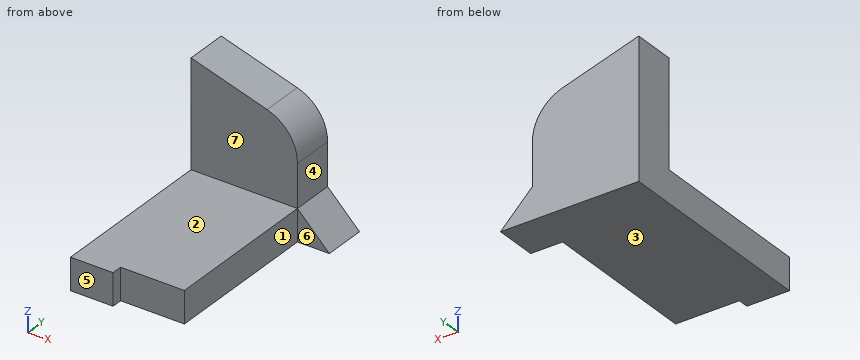
```python
from build123d import *

# Parameters (mm, degrees)
F1_DEPTH = 15
F3_DEPTH = 20
F4_R     = 20
F6_DEPTH = 20


with BuildPart() as f1:
    # F0 (on Top) → F1 (new body)
    with BuildSketch(Plane.XY):
        Polygon((0, 100), (0, 0), (20, 0), (20, 5), (50, 5), (50, 100), align=None)
    extrude(amount=F1_DEPTH)

    # F2 (on face) → F3 (join)
    with BuildSketch(Plane(origin=(0, 100, 0), x_dir=(-1, 0, 0), z_dir=(0, 1, 0))):
        Polygon((-50, 15), (0, 15), (0, 65), (-50, 50), align=None)
    extrude(amount=-F3_DEPTH)

    # F4
    f4_edges = [f1.edges().sort_by_distance(p)[0] for p in [
        (50, 90, 50),
    ]]
    fillet(f4_edges, radius=F4_R)

    # F5 (on face) → F6 (join)
    with BuildSketch(Plane(origin=(0, 100, 0), x_dir=(-1, 0, 0), z_dir=(0, 1, 0))):
        Polygon((-65, 0), (-50, 0), (-50, 15), align=None)
    extrude(amount=-F6_DEPTH)


solid = f1.part
```
For this review, take the finished solid that the model builds, in its own axes (mm). Face numbers are marked on the shaded views. A direction names the side the tool comes from. Coordinates: 2 decimals unless noted, no trailing zeros. Write each loop counter-clockwise with the first axis right and the second up, starting at its lowest first coordinate (ties: lowest second). Pieces come first, ordered by that corner, then holes. Notation, with made-up numbers: (62.5, 11) - (106.5, 11) arc R21 ccw to (106.5, 23) - close; hole circle Ø4 at (-32.5, 40.25). An arc over 180 degrees is marked (long way). Put each result on its own line as item: value.
1. Add section D-D, the plane x = 34. Give the boundary of the cut face in (y, z).
Values found:
outline: (5, 0) - (100, 0) - (100, 54.8) - (80, 54.8) - (80, 15) - (5, 15) - close
2. Wall thickness on probe 1 along Y at (x, z) = (22.5, 28.5); probe 2 along Z at (x, y) = (33, 72); probe 3 along X at (y, z) = (81, 31.5): over which ranges is each line inside the solid? List them lowest first.
Values found:
probe 1: 80 to 100
probe 2: 0 to 15
probe 3: 0 to 50
3. Add section C-C, the plane y = 39. Give the boundary of the cut face in (x, z), then the cut area to 3 significant figures.
Values found:
outline: (0, 0) - (50, 0) - (50, 15) - (0, 15) - close
area: 750 mm²
4. For pin 1 (16 mm diameter, centred on y = 92, z = 21.5, fed in from +X); pin 2 (1.5 mm diameter, centred on y = 3.5, z = 11, fed in from +X); pin 3 (8 mm diameter, centred on x = 13.5, y = 58.5, fed in from +Z), all flat-tipped, find the tip position at first contact; note any pin that passes through.
Values found:
pin 1: x = 51.5
pin 2: x = 20
pin 3: z = 15
5. Add section A-A, the plane z = 4. Give the boundary of the cut face in (x, y).
Values found:
outline: (0, 0) - (20, 0) - (20, 5) - (50, 5) - (50, 80) - (61, 80) - (61, 100) - (0, 100) - close
6. Mouldability with a two-part tool opening along Z and no side actions: class the marked faces 1, 2 and 3 as released by +Z, released by -Z, zero draft, split by the parting line, or undercut.
Values found:
face 1: zero draft
face 2: released by +Z
face 3: released by -Z
7. Machinability: for the marked faces 4, 5, 6 and 7, which of the approach directions +Z, -Z, +X, -X, +Y, -Y give a long, thin tool a straight path to every point of the face, cutting with its end or side? Answer none if there is none.
Values found:
face 4: +Z, +X, +Y, -Y
face 5: +Z, -Z, +X, -X, -Y
face 6: +Z, -Z, +X, -Y
face 7: +Z, +X, -X, -Y
8. Add section B-B, the plane x = 4. Give the boundary of the cut face in (y, z).
Values found:
outline: (0, 0) - (100, 0) - (100, 63.8) - (80, 63.8) - (80, 15) - (0, 15) - close
